Source: three-view drawing plus pictorial views. Frame: mm from the lowest corner of the part. Give positions to 0.01 mm unless a question says otherwise; leave off trailing zeros. Write each loop counter-clockwise with the first axis right and the second up, starting at its lowest first coordinate (ties: lowest second). Pieces come first, ordered by that corner, then holes. Notation, with made-up numbers: (-20, -2.5) - (19, -2.5) arc R28 ccw to (19, 24.5) - close; hole circle Ø10 at (5, 80). An arc over 180 degrees is marked (long way). One line per question, with ' | ' between items. Start each with the question number.
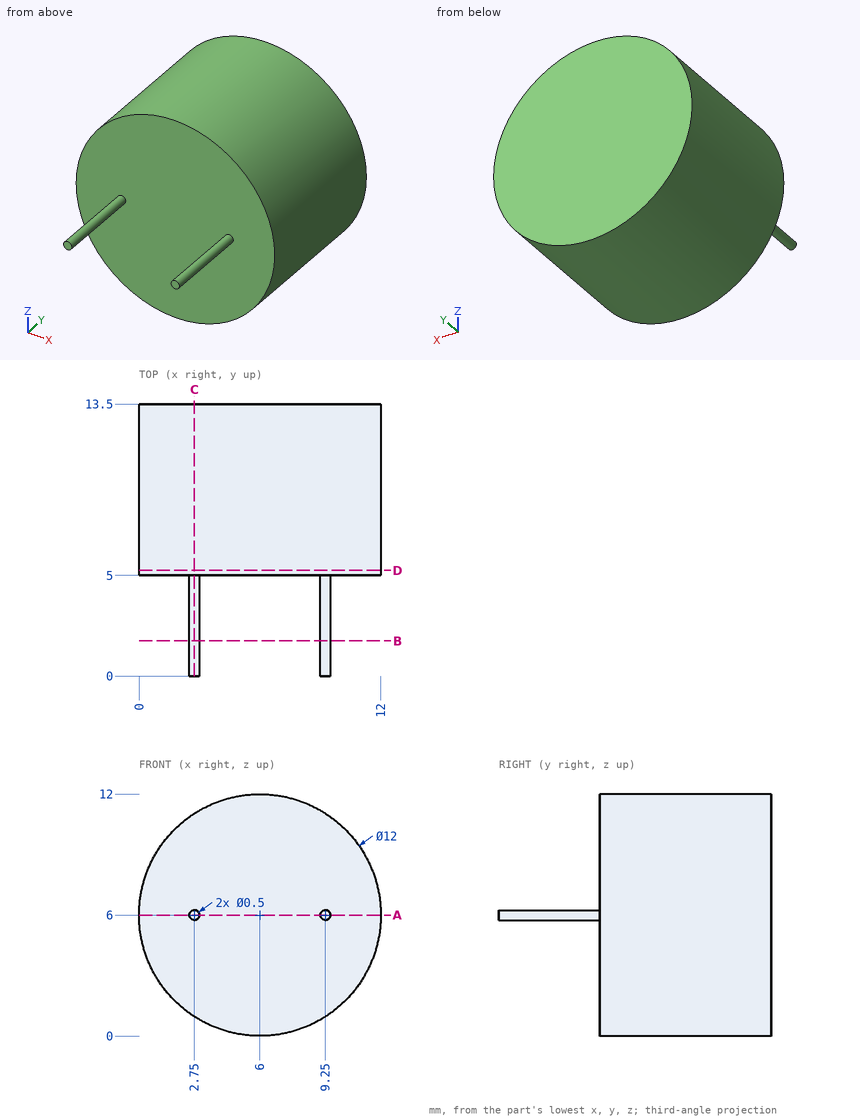
1) Section B-B, the plane y = 1.75. Output: boundary loops of the cut face in (x, z).
2) Section A-A, the plane z = 6. Output: boundary loops of the cut face in (x, y), plus the area to 3 significant figures.
3) Line query: L1, parallel to Y at x = 3.5, z = 9.75; L2, parallel to Z at x = 2.75, y = 1.5; L3, parallel to Z at x = 2, y = 6. Output: solid intervals per line, ascending.
4) Section D-D, the plane y = 5.25. Output: boundary loops of the cut face in (x, z), plus the area to 3 significant figures.
5) First-contact query: pin 1 Ø1 at (x, y) = (10, 11.5) entering from -Z; pin 2 Ø1 at (y, z) = (3, 5.5) entering from -X; pin 3 Ø5 at (x, y) = (9, 1.5) entering from -Z. Flat tips, straight axial feed; report the tip coordinate or a pass-through.
6) Section C-C, the plane x = 2.75. Output: boundary loops of the cut face in (y, z).
Answer key:
1) outline: circle Ø0.5 at (2.75, 6); circle Ø0.5 at (9.25, 6)
2) outline: (0, 5) - (2.5, 5) - (2.5, 0) - (3, 0) - (3, 5) - (9, 5) - (9, 0) - (9.5, 0) - (9.5, 5) - (12, 5) - (12, 13.5) - (0, 13.5) - close | area: 107 mm^2
3) L1: 5 to 13.5 | L2: 5.75 to 6.25 | L3: 1.53 to 10.47
4) outline: circle Ø12 at (6, 6) | area: 113 mm^2
5) pin 1: z = 1.13 | pin 2: x = 2.5 | pin 3: z = 5.75
6) outline: (0, 5.75) - (5, 5.75) - (5, 0.96) - (13.5, 0.96) - (13.5, 11.04) - (5, 11.04) - (5, 6.25) - (0, 6.25) - close
